The model under review builds one solid part; all positions refer to its coordinate system, in mm. A direction names the side the tool comes from. Coordinates: 2 decimals unless noted, no trailing zeros. Order: outer loops, then holes, each group sorted by start corner. A loop starts at its lowest first (then second) coordinate and runs counter-clockwise, first axis right, second up.
```python
from build123d import *

# Parameters (mm, degrees)
SKETCH084_W     = 50.8
SKETCH084_H     = 30.6
PAD021_DEPTH    = 2.5
SKETCH085_R     = 1.6
POCKET071_DEPTH = 2.501
SKETCH086_W     = 50.8
SKETCH086_H     = 6
PAD022_DEPTH    = 19.27
SKETCH087_R     = 6.585
POCKET072_DEPTH = 5
SKETCH088_R     = 2.75
POCKET073_DEPTH = 4
SKETCH089_R     = 5.25
POCKET074_DEPTH = 10.301
CHAMFER013_SIZE = 1.5
FILLET002_R     = 1
FILLET003_R     = 10


with BuildPart() as part:
    # Sketch084 → Pad021 (new body)
    with BuildSketch(Plane.XY):
        Rectangle(SKETCH084_W, SKETCH084_H)
    extrude(amount=PAD021_DEPTH)

    # Sketch085 (on Face5 of Pad021) → Pocket071 (cut, through all)
    with BuildSketch(Plane(origin=(0, 0, 0), x_dir=(1, 0, 0), z_dir=(0, 0, -1))):
        with Locations((-19, 10.775)):
            Circle(SKETCH085_R)
        with Locations((19, 10.775)):
            Circle(SKETCH085_R)
        with Locations((19, -10.8)):
            Circle(SKETCH085_R)
        with Locations((-19, -10.8)):
            Circle(SKETCH085_R)
    extrude(amount=-POCKET071_DEPTH, mode=Mode.SUBTRACT)

    # Sketch086 (on Face4 of Pocket071) → Pad022 (join)
    with BuildSketch(Plane(origin=(0, 0, 0), x_dir=(1, 0, 0), z_dir=(0, 0, -1))):
        with Locations((0, -3)):
            Rectangle(SKETCH086_W, SKETCH086_H)
    extrude(amount=PAD022_DEPTH)

    # Sketch087 (on Face12 of Pad022) → Pocket072 (cut)
    with BuildSketch(Plane.XZ):
        with Locations((-12.9, -9.685)):
            Circle(SKETCH087_R)
    extrude(amount=-POCKET072_DEPTH, mode=Mode.SUBTRACT)

    # Sketch088 (on Face12 of Pocket072) → Pocket073 (cut)
    with BuildSketch(Plane.XZ):
        with Locations((19.9, -9.685)):
            Circle(SKETCH088_R)
    extrude(amount=-POCKET073_DEPTH, mode=Mode.SUBTRACT)

    # Sketch089 (on Face20 of Pocket073) → Pocket074 (cut, through all)
    with BuildSketch(Plane.XZ.offset(-5)):
        with Locations((-12.9, -9.685)):
            Circle(SKETCH089_R)
    extrude(amount=-POCKET074_DEPTH, mode=Mode.SUBTRACT)

    # Chamfer013
    chamfer013_edges = [part.edges().sort_by_distance(p)[0] for p in [
        (-20.6, -10.775, 0),
        (17.4, -10.775, 0),
        (17.4, 10.8, 0),
        (-20.6, 10.8, 0),
    ]]
    chamfer(chamfer013_edges, length=CHAMFER013_SIZE)

    # Fillet002
    fillet002_edges = [part.edges().sort_by_distance(p)[0] for p in [
        (-19.485, 0, -9.685),
        (17.15, 0, -9.685),
    ]]
    fillet(fillet002_edges, radius=FILLET002_R)

    # Fillet003
    fillet003_edges = [part.edges().sort_by_distance(p)[0] for p in [
        (-25.4, 3, -19.27),
        (25.4, 3, -19.27),
    ]]
    fillet(fillet003_edges, radius=FILLET003_R)


solid = part.part
```
(1) We need section C-C, the plane x = 8.5. Write out the cut boundary in (y, z), and give its area (3 significant figures).
A:
outline: (-15.3, 0) - (0, 0) - (0, -19.27) - (6, -19.27) - (6, 0) - (15.3, 0) - (15.3, 2.5) - (-15.3, 2.5) - close
area: 192 mm2
(2) Draft analysis for pull direction Z (two halves, no side actions). For faces 4 (the face through (-25.4, 1, -1)), 5 (the face through (0, -8, 0)), 6 (the face through (-6.62, 2.97, -7.71)), 7 (the face through (-18, 5, -12)), state which applies: released by +Z, released by -Z, zero draft, split by the parting line, or undercut.
A:
face 4: zero draft
face 5: released by -Z
face 6: undercut
face 7: undercut
(3) We need section A-A, the plane y = 10.8. Write out the cut boundary in (x, z), and give its area (4 significant figures).
A:
outline: (-25.4, 0) - (-22.1, 0) - (-20.6, 1.5) - (-20.6, 2.5) - (-25.4, 2.5) - close; (-17.4, 1.5) - (-15.9, 0) - (15.9, 0) - (17.4, 1.5) - (17.4, 2.5) - (-17.4, 2.5) - close; (20.6, 1.5) - (22.1, 0) - (25.4, 0) - (25.4, 2.5) - (20.6, 2.5) - close
area: 106.5 mm2
(4) Wall thickness on probe 1 along X at (y, z) = (10.8, 2.2); probe 2 along Y at (x, z) = (-19, 2) (3 decimals); probe 3 along Z at (x, y) = (-12.9, 5.35) (3 decimals): over which ranges is each line inside the solid? List them lowest first.
A:
probe 1: x = -25.4 to -20.6, -17.4 to 17.4, 20.6 to 25.4
probe 2: y = -15.3 to -12.375, -9.175 to 9.2, 12.4 to 15.3
probe 3: z = -19.27 to -14.935, -4.435 to 2.5
(5) We need section D-D, the plane y = 2. Write out the cut boundary in (x, z) (3 decimals), and give its area (3 significant figures).
A:
outline: (-25.4, -9.27) arc R10 ccw to (-15.4, -19.27) - (15.4, -19.27) arc R10 ccw to (25.4, -9.27) - (25.4, 2.5) - (-25.4, 2.5) - close; hole circle Ø13.17 at (-12.9, -9.685); hole circle Ø5.5 at (19.9, -9.685)
area: 903 mm2
(6) We need section B-B, the plane x = -12.9. Write out the cut boundary in (y, z) (3 decimals).
A:
outline: (-15.3, 0) - (0, 0) - (0, -2.1) arc R1 ccw to (1, -3.1) - (5, -3.1) - (5, -4.435) - (6, -4.435) - (6, 0) - (15.3, 0) - (15.3, 2.5) - (-15.3, 2.5) - close; (0, -19.27) - (6, -19.27) - (6, -14.935) - (5, -14.935) - (5, -16.27) - (1, -16.27) arc R1 ccw to (0, -17.27) - close
(7) Machinability: for faces 1 (the face through (17.73, 11.77, 1.99)), 2 (the face through (0, 6, -10)), 3 (the face through (20, 4, -10)), which of the approach directions +Z, -Z, +X, -X, +Y, -Y give a long, thin tool a straight path to every point of the face, cutting with its end or side? Answer none if there is none.
A:
face 1: +Z, -Z
face 2: -Z, +X, -X, +Y
face 3: -Y
(8) For pin 1 Ø4 at (x, z) = (-11.5, -10) entering from -Y; pin 2 Ø8 at (x, z) = (-13.5, -12.5) entering from +Y; pin 3 Ø10 at (x, y) = (4.5, -9) entering from -Z; pin 4 Ø4 at (x, y) = (19, -10.775) entering from -Z, all flat-tipped, find the tip position at first contact; note any pin that passes through.
A:
pin 1: passes through
pin 2: stops at y = 6
pin 3: stops at z = 0
pin 4: stops at z = 1.1
